from build123d import *

# Parameters (mm, degrees)
ESBO_O1_W                = 138
ESBO_O1_H                = 63
RESSALTO_EXTRUS_O1_DEPTH = 4
ESBO_O2_W                = 8
ESBO_O2_H                = 63
RESSALTO_EXTRUS_O2_DEPTH = 2
ESBO_O3_W                = 8
ESBO_O3_H                = 46.7
RESSALTO_EXTRUS_O3_DEPTH = 5
ESBO_O4_R                = 1.65
CORTE_EXTRUS_O1_DEPTH    = 77.643655967
CORTE_EXTRUS_O2_DEPTH    = 3.3
FILETE1_R                = 7


with BuildPart() as part:
    # Esboço1 → Ressalto-extrusão1 (new body)
    with BuildSketch(Plane.XY):
        Rectangle(ESBO_O1_W, ESBO_O1_H)
    extrude(amount=RESSALTO_EXTRUS_O1_DEPTH)

    # Esboço2 → Ressalto-extrusão2 (add)
    with BuildSketch(Plane.XY.offset(4)):
        with Locations((65, 0)):
            Rectangle(ESBO_O2_W, ESBO_O2_H)
        with Locations((-65, 0)):
            Rectangle(ESBO_O2_W, ESBO_O2_H)
    extrude(amount=RESSALTO_EXTRUS_O2_DEPTH)

    # Esboço3 → Ressalto-extrusão3 (add)
    with BuildSketch(Plane.XY.offset(6)):
        with Locations((65, 0)):
            Rectangle(ESBO_O3_W, ESBO_O3_H)
        with Locations((-65, 0)):
            Rectangle(ESBO_O3_W, ESBO_O3_H)
    extrude(amount=RESSALTO_EXTRUS_O3_DEPTH)

    # Esboço4 → Corte-extrusão1 (cut, through all)
    with BuildSketch(Plane(origin=(0, 0, 0), x_dir=(-1, 0, 0), z_dir=(0, 0, -1))):
        with Locations((65, -13.5)):
            Circle(ESBO_O4_R)
        with Locations((65, 13.5)):
            Circle(ESBO_O4_R)
        with Locations((-65, -9.6)):
            Circle(ESBO_O4_R)
    extrude(amount=-CORTE_EXTRUS_O1_DEPTH, mode=Mode.SUBTRACT)

    # Esboço5 → Corte-extrusão2 (cut)
    with BuildSketch(Plane(origin=(0, 0, 0), x_dir=(-1, 0, 0), z_dir=(0, 0, -1))):
        with BuildLine():
            Line((65, -17), (69, -17))
            Line((69, -17), (69, -10))
            Line((69, -10), (65, -10))
            ThreePointArc((65, -10), (61.5, -13.5), (65, -17))
        make_face()
        with BuildLine():
            Line((65, 10), (69, 10))
            Line((69, 10), (69.148700963, 17))
            Line((69.148700963, 17), (65, 17))
            ThreePointArc((65, 17), (61.5, 13.5), (65, 10))
        make_face()
        with BuildLine():
            Line((-65, -6.1), (-69, -6.1))
            Line((-69, -6.1), (-69, -13.1))
            Line((-69, -13.1), (-65, -13.1))
            ThreePointArc((-65, -13.1), (-61.5, -9.6), (-65, -6.1))
        make_face()
    extrude(amount=-CORTE_EXTRUS_O2_DEPTH, mode=Mode.SUBTRACT)

    # Filete1
    filete1_edges = [part.edges().sort_by_distance(p)[0] for p in [
        (61, 0, 4),
        (-61, 0, 4),
    ]]
    fillet(filete1_edges, radius=FILETE1_R - 0.0001)  # a hair under: the kernel refuses the full size


solid = part.part
Model file for the job. Use its own axes, mm. A direction names the side the tool comes from. Coordinates: 2 decimals unless noted, no trailing zeros. Order: outer loops, then holes, each group sorted by start corner. A loop starts at its lowest first (then second) coordinate and runs counter-clockwise, first axis right, second up. Notation, with made-up numbers: (-11.5, 86.5) -> (12.5, 86.5) arc R14 ccw to (12.5, 105.5) -> close; hole circle Ø5 at (-17, 39.25). An arc over 180 degrees is marked (long way). Return JSON: item names as keys, results as strings. Group by question number.
Item 1: Saw through at A-A on z = 8.5. Write the cut outline in (x, y).
Item 2: Wall check: line 1 along Y through (x, z) = (-65, 8); line 2 along X through (y, z) = (-10, 5); line 3 along Z through (x, y) = (-48, 15). Give the ranges that are in metal, low to high. Write a range as [from, to].
Item 3: Tool access for faces 1 (the flat face through (-64, 27, 6)), 2 (the flat face through (64, -27, 6)), 3 (the flat face through (67, -6.1, 2)), 4 (the flat face through (-67, 17, 2)), 5 (the cylindrical face through (-58.9, 0.4, 6)): list every direction of +Z, -Z, +X, -X, +Y, -Y with a clear straight run to the whole face (end or side of a thin tool).
Item 4: Flat gauge pins, fed straight in: P1, Ø6, axis at x = 4.5, y = -18.5, coming from the +Z side; P2, Ø4, axis at x = 63, y = 28.5, coming from the +Z side; P3, Ø5.5, axis at x = 63, z = 9.5, coming from the -Y side; P4, Ø3, axis at x = 65, y = -9.6, coming from the -Z side. Where does each tip first touch, or does it go through?
Item 5: Saw through at C-C on y = 25. Write the cut outline in (x, z).
Item 6: Saw through at D-D on x = -25. Write the cut outline in (y, z), then the cut area to 3 significant figures.
Item 7: Pull direction Y, two halves, no side cores. Call faces 6 (the cylindrical face through (59, 0.4, 6.1)), 7 (the flat face through (65, 23.35, 8)), 8 (the cylindrical face through (-63.35, 13.57, 7.1)), 9 (the flat face through (-65, -23.35, 8)): pulls with the +Y half, pulls with the -Y half, needs draft (parallel to the pull), parting line crosses it, or undercut.
Values found:
{
 "1": {"outline": "(-69, -23.35) -> (-60.54, -23.35) -> (-60.54, 23.35) -> (-69, 23.35) -> close; (60.54, -23.35) -> (69, -23.35) -> (69, 23.35) -> (60.54, 23.35) -> close; hole circle Ø3.3 at (-65, -13.5); hole circle Ø3.3 at (-65, 13.5); hole circle Ø3.3 at (65, -9.6)"},
 "2": {"line 1": "y = [-23.35, -15.15], [-11.85, 11.85], [15.15, 23.35]", "line 2": "x = [-69, -57.61], [57.61, 63.4], [66.6, 69]", "line 3": "z = [0, 4]"},
 "3": {"face 1": "+Z, +X, -X, +Y", "face 2": "+Z, +X, -X, -Y", "face 3": "-Z, +X", "face 4": "-Z, -X", "face 5": "+Z, +Y, -Y"},
 "4": {"P1": "stops at z = 4", "P2": "stops at z = 6", "P3": "stops at y = -23.35", "P4": "passes through"},
 "5": {"outline": "(-69, 0) -> (69, 0) -> (69, 6) -> (58.9, 6) arc R7 cw to (54, 4) -> (-54, 4) arc R7 cw to (-58.9, 6) -> (-69, 6) -> close"},
 "6": {"outline": "(-31.5, 0) -> (31.5, 0) -> (31.5, 4) -> (-31.5, 4) -> close", "area": "252 mm2"},
 "7": {"face 6": "needs draft", "face 7": "pulls with the +Y half", "face 8": "undercut", "face 9": "pulls with the -Y half"}
}
